Can you work these out from the model? Positions are in its coordinate system, mm. Face numbers are marked on the shaded views. A direction names the side the tool comes from. Round coordinates to 2 decimals unless told otherwise and drop trailing zeros. Loops run counter-clockwise (first coordinate to the right, second up) from the corner with the lowest first, then second, coordinate; pieces in that order, holes last. Notation, with made-up numbers: (17.25, 21.5) -> (35.25, 21.5) arc R13 ccw to (35.25, 37.5) -> close; hole circle Ø6 at (32, 30). An arc over 180 degrees is marked (long way). Use a Markdown table: item, result.
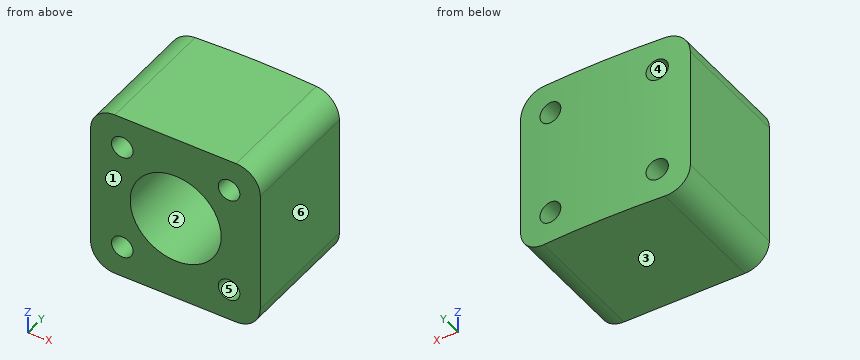
from build123d import *

# Parameters (mm, degrees)
BOSS_EXTRUDE1_DEPTH              = 8.89
BOSS_EXTRUDE1_DEPTH_BACK         = 8.89
F_3_8_0_375_DIAMETER_SLOT1_D     = 9.525
F_3_8_0_375_DIAMETER_SLOT1_DEPTH = 9.652
F_3_8_0_375_DIAMETER_SLOT1_TIP   = 2.861598698
TAP_DRILL_FOR_4_40_TAP1_D        = 2.2606
FILLET1_R                        = 2.54


with BuildPart() as part:
    # Sketch1 → Boss-Extrude1 (new, two sides: drawn at the far end of the back side and taken through both)
    with BuildSketch(Plane.XY.offset(-BOSS_EXTRUDE1_DEPTH_BACK)):
        with BuildLine():
            Line((8.853671113, 101.352246104), (8.853671113, 88.534433979))
            Line((8.853671113, 88.534433979), (-8.902635044, 88.534433979))
            Line((-8.902635044, 88.534433979), (-8.902635044, 101.350105765))
            ThreePointArc((-8.902635044, 101.350105765), (-0.024528813, 101.739820854), (8.853671113, 101.352246104))
        make_face()
    extrude(amount=BOSS_EXTRUDE1_DEPTH + BOSS_EXTRUDE1_DEPTH_BACK)

    # 3/8 (0.375) Diameter Slot1
    with Locations(Plane(origin=(0, 88.534433979, 0), x_dir=(-1, 0, 0), z_dir=(0, -1, 0))):
        with Locations((0, 0)):
            Hole(F_3_8_0_375_DIAMETER_SLOT1_D / 2, depth=F_3_8_0_375_DIAMETER_SLOT1_DEPTH)
            with Locations((0, 0, -(F_3_8_0_375_DIAMETER_SLOT1_DEPTH + F_3_8_0_375_DIAMETER_SLOT1_TIP / 2))):  # 118° drill point
                Cone(0, F_3_8_0_375_DIAMETER_SLOT1_D / 2, F_3_8_0_375_DIAMETER_SLOT1_TIP, mode=Mode.SUBTRACT)

    # Tap Drill for #4-40 Tap1 (through all)
    with Locations(Plane(origin=(0, 88.534433979, 0), x_dir=(-1, 0, 0), z_dir=(0, -1, 0))):
        with Locations((-5.588, 5.588), (5.588, 5.588), (5.588, -5.588), (-5.588, -5.588)):
            Hole(TAP_DRILL_FOR_4_40_TAP1_D / 2)

    # Fillet1
    fillet1_edges = [part.edges().sort_by_distance(p)[0] for p in [
        (-8.902635044, 94.942269872, 8.89),
        (8.853671113, 94.943340042, -8.89),
        (8.853671113, 94.943340042, 8.89),
        (-8.902635044, 94.942269872, -8.89),
    ]]
    fillet(fillet1_edges, radius=FILLET1_R)


solid = part.part
1. If we mould it in two halves opening along X, with no side actions, what happens to the marked faces 3, 4, 5 and 6? For each: +X half, -X half, draft (parallel to the pull), parting line (faces both ways), or undercut.
Answer sheet:
| item | result |
|---|---|
| face 3 | draft |
| face 4 | undercut |
| face 5 | undercut |
| face 6 | +X half |
2. I want a section at C-C (z = 7.5). Please give me the cut outline in (x, y).
Answer sheet:
| item | result |
|---|---|
| outline | (-8.63, 88.53) -> (8.58, 88.53) -> (8.58, 101.38) arc R101.6 ccw to (-8.63, 101.37) -> close |
3. I want a section at A-A (y = 94.75). State how many separate pieces and enclosed holes the cut face has, plus the area to 3 significant figures.
Answer sheet:
| item | result |
|---|---|
| separate pieces | 1 |
| enclosed holes | 5 |
| area | 223 mm² |
4. Which directions (+Z, -Z, +X, -X, +Y, -Y) give clear straight access to the entire face, cutting with the end or side of a thin tool? Please do the marked faces 1 and 2.
Answer sheet:
| item | result |
|---|---|
| face 1 | +Z, -Z, +X, -X, -Y |
| face 2 | -Y |
5. I want a section at B-B (x = -5.75). Please give me the cut outline in (y, z).
Answer sheet:
| item | result |
|---|---|
| outline | (88.53, -8.89) -> (101.58, -8.89) -> (101.58, -6.71) -> (88.53, -6.71) -> close; (88.53, -4.47) -> (101.58, -4.47) -> (101.58, 4.47) -> (88.53, 4.47) -> close; (88.53, 6.71) -> (101.58, 6.71) -> (101.58, 8.89) -> (88.53, 8.89) -> close |
6. I need wall thicknesses on line 1 (X direction, y = 93, z = 5.5); line 2 (Z direction, x = 0, y = 90.5); line 3 (Z direction, x = -5.5, y = 90). Which ranges of each line are inside material? Lowest first, please.
Answer sheet:
| item | result |
|---|---|
| line 1 | x = -8.9 to -6.71, -4.46 to 4.46, 6.71 to 8.85 |
| line 2 | z = -8.89 to -4.76, 4.76 to 8.89 |
| line 3 | z = -8.89 to -6.71, -4.46 to 4.46, 6.71 to 8.89 |
7. Will these pins go through, and if not, where does the flat tip stop? pin 1 Ø1.5 at (x, z) = (3.5, -1.5) entering from -Y; pin 2 Ø3.5 at (x, z) = (-5.588, 5.588) entering from +Y; pin 3 Ø5.5 at (x, z) = (0, 0) entering from -Y.
Answer sheet:
| item | result |
|---|---|
| pin 1 | stops at y = 98.31 |
| pin 2 | stops at y = 101.67 |
| pin 3 | stops at y = 99.4 |
